```python
from build123d import *

# Parameters (mm, degrees)
SKETCH1_W           = 14
SKETCH1_H           = 14
SKETCH1_R           = 1.75
BOSS_EXTRUDE1_DEPTH = 3
SKETCH2_W           = 14
SKETCH2_H           = 17
SKETCH2_R           = 1.65
BOSS_EXTRUDE2_DEPTH = 3
BOSS_EXTRUDE3_DEPTH = 2
BOSS_EXTRUDE4_DEPTH = 2


with BuildPart() as part:
    # Sketch1 → Boss-Extrude1 (new body)
    with BuildSketch(Plane(origin=(0, 0, 0), x_dir=(1, 0, 0), z_dir=(0, 1, 0))):
        with Locations((-7, 7)):
            Rectangle(SKETCH1_W, SKETCH1_H)
        with Locations((-7, 7)):
            Circle(SKETCH1_R, mode=Mode.SUBTRACT)
    extrude(amount=BOSS_EXTRUDE1_DEPTH)

    # Sketch2 → Boss-Extrude2 (add)
    with BuildSketch(Plane(origin=(0, 0, 0), x_dir=(0, 0, -1), z_dir=(1, 0, 0))):
        with Locations((7, 8.5)):
            Rectangle(SKETCH2_W, SKETCH2_H)
        with Locations((7, 10)):
            Circle(SKETCH2_R, mode=Mode.SUBTRACT)
    extrude(amount=BOSS_EXTRUDE2_DEPTH)

    # Sketch3 → Boss-Extrude3 (add)
    with BuildSketch(Plane.XY):
        Polygon((0, 3), (0, 17), (-14, 3), align=None)
    extrude(amount=-BOSS_EXTRUDE3_DEPTH)

    # Sketch4 → Boss-Extrude4 (add)
    with BuildSketch(Plane(origin=(0, 0, -14), x_dir=(-1, 0, 0), z_dir=(0, 0, -1))):
        Polygon((0, 3), (14, 3), (0, 17), align=None)
    extrude(amount=-BOSS_EXTRUDE4_DEPTH)


solid = part.part
```
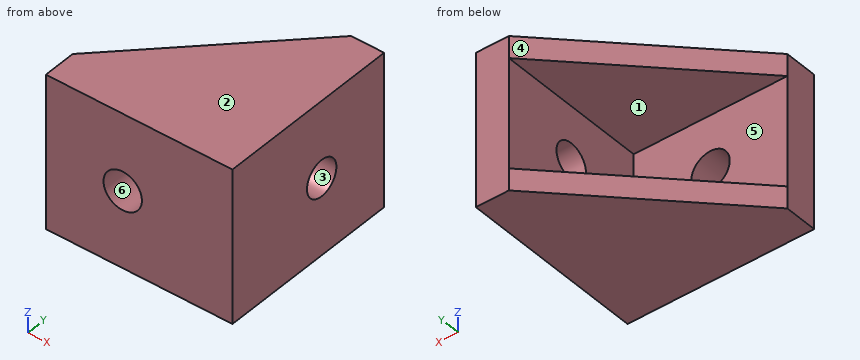
Read the model definition and answer for the solid it produces. Units are mm, in the model's axes. Face numbers are marked on the shaded views. A direction names the side the tool comes from. Give positions to 0.01 mm unless a question says otherwise; leave off trailing zeros. Write each loop counter-clockwise with the first axis right and the second up, starting at its lowest first coordinate (ties: lowest second). Pieces come first, ordered by that corner, then holes. Notation, with made-up numbers: (9, 70.5) - (44, 70.5) arc R17 ccw to (44, 89.5) - close; hole circle Ø6 at (-10.5, -29). An arc over 180 degrees is marked (long way). Write item = value, one per line. Start each with the question number.
Item 1: Find section D-D (y = 10). Give the vertices of the cut face in (x, z), then the cut area to 3 significant figures.
Item 2: Find section C-C (x = -7). Give the vertices of the cut face in (y, z), then the cut area to 3 significant figures.
Item 3: The mould has two halves that part along Z. Classify the marked faces 1, 2, 3 and 4: +Z half, -Z half, draft (parallel to the pull), parting line (faces both ways), or undercut.
Item 4: A tool of negligible diameter and unlimited length cuts with its end or side. For the marked faces 5 and 6, from which of +Z, -Z, +X, -X, +Y, -Y can it reach the whole face along a straight path? Write none if from no direction.
Item 5: Each of these flat-tipped pins is pushed along its axis until it touches: P1, Ø2, axis at y = 11.5, z = -4.5, coming from the -X side; P2, Ø2, axis at y = 10, z = -7, coming from the +X side. Where does it stop, or does it pass through?
Item 6: Find section A-A (z = -7). Give the vertices of the cut face in (x, y), then the cut area to 3 significant figures.
Item 7: Find the intervals of material crossed by probe 1 along Z at (x, y) = (-2.5, 5.5); probe 2 along X at (y, z) = (2, -7); probe 3 along Z at (x, y) = (-7, 0.85), in increasing order. Write a range as [from, to].
Item 8: Find section B-B (y = 4). Give the vertices of the cut face in (x, z).
Response:
q1.outline = (-7, -14) - (3, -14) - (3, -8.65) - (0, -8.65) - (0, -12) - (-7, -12) - close; (-7, -2) - (0, -2) - (0, -5.35) - (3, -5.35) - (3, 0) - (-7, 0) - close
q1.area = 60.1 mm²
q2.outline = (0, -14) - (10, -14) - (10, -12) - (3, -12) - (3, -8.75) - (0, -8.75) - close; (0, -5.25) - (3, -5.25) - (3, -2) - (10, -2) - (10, 0) - (0, 0) - close
q2.area = 59.5 mm²
q3.face_1 = undercut
q3.face_2 = +Z half
q3.face_3 = undercut
q3.face_4 = draft
q4.face_5 = -X, +Y
q4.face_6 = +Y, -Y
q5.P1 = 0
q5.P2 = through
q6.outline = (-14, 0) - (-8.75, 0) - (-8.75, 3) - (-14, 3) - close; (-5.25, 0) - (3, 0) - (3, 8.35) - (0, 8.35) - (0, 3) - (-5.25, 3) - close; (0, 11.65) - (3, 11.65) - (3, 17) - (0, 17) - close
q6.area = 72.6 mm²
q7.probe_1 = [-14, -12], [-2, 0]
q7.probe_2 = [-14, -8.75], [-5.25, 3]
q7.probe_3 = [-14, -8.75], [-5.25, 0]
q8.outline = (-13, -14) - (3, -14) - (3, 0) - (-13, 0) - (-13, -2) - (0, -2) - (0, -12) - (-13, -12) - close
